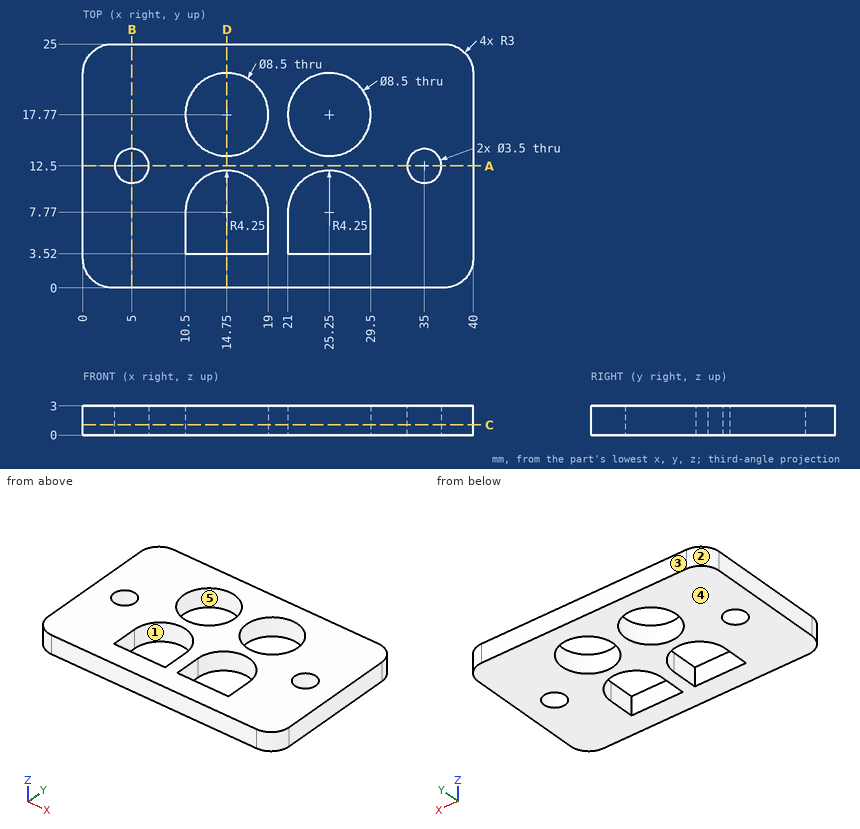
Part print with two shaded views. Sizes in mm from the minimum x, y, z corner. A direction names the side the tool comes from. Round coordinates to 2 decimals unless told otherwise and drop trailing zeros. Order: outer loops, then holes, each group sorted by start corner. A loop starts at its lowest first (then second) coordinate and runs counter-clockwise, first axis right, second up. Notation, with made-up numbers: M 8,-13.75 L 50,-13.75 A15 ccw 50,3.25 Z; hole C 70,79 d7. An arc over 180 degrees is marked long. Answer in a Markdown table with one row per item. Add a question column.
Q1. Pin check, flat tip, straight feed: pin 1 (3 mm diameter, centred on x = 35, y = 12.5, fed in from +Z). Stop position of the tip, or through.
Q2. Cut at A-A on y = 12.5. Give the cut face in (x, z).
Q3. Mould opens along Y. For the marked faces 3, 4 and 5 say: +Y half, -Y half, draft (parallel to the pull), parting line (faces both ways), or undercut.
Q4. Cut at D-D on x = 14.75. Give the cut face in (y, z).
Q5. Wall check: L1, parallel to Y at x = 25.25, z = 2.2; L2, parallel to X at y = 18.5, z = 0.6; L3, parallel to X at y = 15, z = 1.4. Give the ranges that are in metal, low to high. Write a range as from..to.
Q6. 3-axis set-ups, long thin cutter, end or side, ignore diameter. For the marked faces 1 and 2: which of +Z, -Z, +X, -X, +Y, -Y reach the whole face in a straight line?
Q7. Cut at B-B on x = 5. Give the cut face in (y, z), and give its area (3 significant figures).
Q8. Cut at C-C on z = 1.05. Give the cut face in (x, y), and give its area (3 significant figures).
Established:
| question | item | result |
|---|---|---|
| 1 | pin 1 | passes through |
| 2 | outline | M 0,0 L 3.25,0 L 3.25,3 L 0,3 Z; M 6.75,0 L 33.25,0 L 33.25,3 L 6.75,3 Z; M 36.75,0 L 40,0 L 40,3 L 36.75,3 Z |
| 3 | face 3 | +Y half |
| 3 | face 4 | draft |
| 3 | face 5 | undercut |
| 4 | outline | M 0,0 L 3.52,0 L 3.52,3 L 0,3 Z; M 12.02,0 L 13.52,0 L 13.52,3 L 12.02,3 Z; M 22.02,0 L 25,0 L 25,3 L 22.02,3 Z |
| 5 | L1 | y = 0..3.52, 12.02..13.52, 22.02..25 |
| 5 | L2 | x = 0..10.56, 18.94..21.06, 29.44..40 |
| 5 | L3 | x = 0..11.53, 17.97..22.03, 28.47..40 |
| 6 | face 1 | +Z, -Z |
| 6 | face 2 | +Z, -Z, -X, +Y |
| 7 | outline | M 0,0 L 10.75,0 L 10.75,3 L 0,3 Z; M 14.25,0 L 25,0 L 25,3 L 14.25,3 Z |
| 7 | area | 64.5 mm2 |
| 8 | outline | M 0,3 A3 ccw 3,0 L 37,0 A3 ccw 40,3 L 40,22 A3 ccw 37,25 L 3,25 A3 ccw 0,22 Z; hole C 5,12.5 d3.5; hole M 10.5,3.52 L 19,3.52 L 19,7.77 A4.25 ccw 10.5,7.77 Z; hole C 14.75,17.77 d8.5; hole M 21,3.52 L 29.5,3.52 L 29.5,7.77 A4.25 ccw 21,7.77 Z; hole C 25.25,17.77 d8.5; hole C 35,12.5 d3.5 |
| 8 | area | 731 mm2 |
